from build123d import *

# Parameters (mm, degrees)
CROQUIS1_R              = 4
CROQUIS1_R_2            = 1.5
SALIENTE_EXTRUIR1_DEPTH = 7
CROQUIS3_W              = 4
CROQUIS3_H              = 3.585282108
SALIENTE_EXTRUIR2_DEPTH = 49
CROQUIS4_R              = 4
CROQUIS4_R_2            = 1.5
SALIENTE_EXTRUIR3_DEPTH = 8
NERVIO1_REACH           = 55.61
CROQUIS6_WALL_W         = 119.09857021
CROQUIS6_WALL_H         = 1


with BuildPart() as part:
    # Croquis1 → Saliente-Extruir1 (new body)
    with BuildSketch(Plane.XY):
        with Locations((0, -10)):
            Circle(CROQUIS1_R)
        with Locations((0, -10)):
            Circle(CROQUIS1_R_2, mode=Mode.SUBTRACT)
    extrude(amount=SALIENTE_EXTRUIR1_DEPTH)

    # Croquis3 → Saliente-Extruir2 (add)
    with BuildSketch(Plane.ZY):
        with Locations((2, -10)):
            Rectangle(CROQUIS3_W, CROQUIS3_H)
    extrude(amount=-SALIENTE_EXTRUIR2_DEPTH)

    # Croquis4 → Saliente-Extruir3 (add)
    with BuildSketch(Plane.XY.offset(7)):
        with Locations((49, -10)):
            Circle(CROQUIS4_R)
        with Locations((49, -10)):
            Circle(CROQUIS4_R_2, mode=Mode.SUBTRACT)
    extrude(amount=-SALIENTE_EXTRUIR3_DEPTH)

    # Croquis6 wall → Nervio1 (add, up to next)
    with BuildSketch(Plane(origin=(42.914213562, -10, -0.5), x_dir=(-0.994863752618, 0, 0.1012230889), z_dir=(-0.1012230889, 0, -0.994863752618)), mode=Mode.PRIVATE) as nervio1_sk1:
        Rectangle(CROQUIS6_WALL_W, CROQUIS6_WALL_H)
    nervio1_tool1 = extrude(nervio1_sk1.sketch, amount=-NERVIO1_REACH, mode=Mode.PRIVATE) - part.part
    add(nervio1_tool1.solids().sort_by_distance((42.914213562, -10, -0.5))[0])


solid = part.part
Here's how the part is built. I have some questions about the finished solid (model axes, mm). A direction names the side the tool comes from. Give positions to 0.01 mm unless a question says otherwise; leave off trailing zeros. Order: outer loops, then holes, each group sorted by start corner. A loop starts at its lowest first (then second) coordinate and runs counter-clockwise, first axis right, second up. Notation, with made-up numbers: M 67.25,24.5 L 87.25,24.5 A24 cw 87.25,56.5 Z; hole C 39.5,-15.5 d10. An arc over 180 degrees is marked long. Answer as a JSON object with one key per item and string values. Group by question number.
1) Suppose I cut it at D-D, the plane x = 1. Write out the boundary of the cut face in (y, z), plus the area to 3 significant figures.
2) I'm going to push flat-ended pins straight in: pin 1 Ø2.5 at (x, y) = (0, -10) entering from -Z; pin 2 Ø0.8 at (x, z) = (41.5, -0.5) entering from +Y; pin 3 Ø3 at (x, z) = (8.5, 1.5) entering from +Y; pin 4 Ø1.6 at (x, y) = (48, -10) entering from +Z. Where does each tip first touch, or does it pass through?
3) We'd pull the mould along X, two halves only. Please class faces 4 (the flat face through (24, -10, 4)), 5 (the flat face through (49, -12, 7)), 6 (the flat face through (41.565, -9.993, -0.363)): pulls with the +X half, pulls with the -X half, needs draft (parallel to the pull), parting line crosses it, or undercut.
4) Suppose I cut it at C-C, the plane y = -10. Write out the boundary of the cut face in (x, z), plus the area to 3 significant figures.
5) Please list where these lines run through material, in increasing order: L1, parallel to X at y = -10, z = 5; L2, parallel to Y at x = 49, z = 5.75; L3, parallel to Y at x = 16.5, z = 3.75. Write a range as [from, to].
6) On a 3-axis mill with a long thin cutter (end or side, diameter ignored), from which of +Z, -Z, +X, -X, +Y, -Y can I reach the whole of each face in a straight line? I mean faces 1 (the flat face through (24, -11.793, 2)), 2 (the flat face through (49, -10, 2)), 3 (the cylindrical face through (-1.5, -9.93, 4.23)). Say none if no direction works.
7) Suppose I cut it at A-A, the plane z = 3.25. Write out the boundary of the cut face in (x, y).
8) Suppose I cut it at B-B, the plane y = -6.75. Write out the boundary of the cut face in (x, z).
Results found:
{
 "1": {"outline": "M -13.87,0 L -6.13,0 L -6.13,7 L -8.88,7 L -8.88,4 L -11.12,4 L -11.12,7 L -13.87,7 Z", "area": "47.5 mm²"},
 "2": {"pin 1": "z = 0", "pin 2": "y = -9.5", "pin 3": "y = -8.21", "pin 4": "z = 7"},
 "3": {"face 4": "undercut", "face 5": "needs draft", "face 6": "pulls with the -X half"},
 "4": {"outline": "M -4,0 L -1.5,0 L -1.5,7 L -4,7 Z; M 0,0 L 38,0 L 45,-0.71 L 45,-1 L 47.5,-1 L 47.5,0 L 49,0 L 49,4 L 47.5,4 L 47.5,7 L 45,7 L 45,4 L 4,4 L 4,7 L 1.5,7 L 1.5,4 L 0,4 Z; M 50.5,-1 L 53,-1 L 53,7 L 50.5,7 Z", "area": "253 mm²"},
 "5": {"L1": "[-4, -1.5], [1.5, 4], [45, 47.5], [50.5, 53]", "L2": "[-14, -11.5], [-8.5, -6]", "L3": "[-11.79, -8.21]"},
 "6": {"face 1": "+Z, -Z, -Y", "face 2": "+Z, -Z", "face 3": "+Z"},
 "7": {"outline": "M 3.58,-11.79 L 45.42,-11.79 A4 ccw long 45.42,-8.21 L 3.58,-8.21 A4 ccw long Z; hole M 0,-11.5 L 0,-8.5 A1.5 ccw Z; hole M 49,-11.5 A1.5 ccw 49,-8.5 Z"},
 "8": {"outline": "M -2.33,0 L 2.33,0 L 2.33,7 L -2.33,7 Z; M 46.67,-1 L 51.33,-1 L 51.33,7 L 46.67,7 Z"}
}
